from build123d import *

# Parameters (mm, degrees)
SKETCH_1_R          = 1.75
SKETCH_1_R_2        = 7.5
EXTRUDE_1_DEPTH     = 5
SKETCH_1_3_R        = 7.5
SKETCH_1_3_R_2      = 4
EXTRUDE_2_DEPTH     = 24
SKETCH_2_R          = 3
CUT_EXTRUDE_1_DEPTH = 3.1
CHAMFER_1_SIZE      = 0.5
CHAMFER_2_SIZE      = 0.5
FILLET_1_R          = 0.5


with BuildPart() as part:
    # 草图1 → 凸台-拉伸1 (new body)
    with BuildSketch(Plane(origin=(0, 0, 0), x_dir=(1, 0, 0), z_dir=(0, 1, 0))):
        with BuildLine():
            ThreePointArc((-12.5, -9.987492178), (-11.313708499, -11.313708499), (-9.987492178, -12.5))
            Line((-9.987492178, -12.5), (9.987492178, -12.5))
            ThreePointArc((9.987492178, -12.5), (11.313708499, -11.313708499), (12.5, -9.987492178))
            Line((12.5, -9.987492178), (12.5, 9.987492178))
            ThreePointArc((12.5, 9.987492178), (11.313708499, 11.313708499), (9.987492178, 12.5))
            Line((9.987492178, 12.5), (-9.987492178, 12.5))
            ThreePointArc((-9.987492178, 12.5), (-11.313708499, 11.313708499), (-12.5, 9.987492178))
            Line((-12.5, 9.987492178), (-12.5, -9.987492178))
        make_face()
        with Locations((-8.485281374, -8.485281374)):
            Circle(SKETCH_1_R, mode=Mode.SUBTRACT)
        with Locations((8.485281374, -8.485281374)):
            Circle(SKETCH_1_R, mode=Mode.SUBTRACT)
        with Locations((-8.485281374, 8.485281374)):
            Circle(SKETCH_1_R, mode=Mode.SUBTRACT)
        Circle(SKETCH_1_R_2, mode=Mode.SUBTRACT)
        with Locations((8.485281374, 8.485281374)):
            Circle(SKETCH_1_R, mode=Mode.SUBTRACT)
    extrude(amount=EXTRUDE_1_DEPTH)

    # 草图1<3> → 凸台-拉伸2 (add)
    with BuildSketch(Plane(origin=(0, 0, 0), x_dir=(1, 0, 0), z_dir=(0, 1, 0))):
        Circle(SKETCH_1_3_R)
        Circle(SKETCH_1_3_R_2, mode=Mode.SUBTRACT)
    extrude(amount=EXTRUDE_2_DEPTH)

    # 草图2 → 切除-拉伸1 (cut)
    with BuildSketch(Plane.XZ):
        with Locations((-8.485281374, 8.485281374)):
            Circle(SKETCH_2_R)
        with Locations((8.485281374, 8.485281374)):
            Circle(SKETCH_2_R)
        with Locations((8.485281374, -8.485281374)):
            Circle(SKETCH_2_R)
        with Locations((-8.485281374, -8.485281374)):
            Circle(SKETCH_2_R)
    extrude(amount=-CUT_EXTRUDE_1_DEPTH, mode=Mode.SUBTRACT)

    # 倒角1
    chamfer_1_edges = [part.edges().sort_by_distance(p)[0] for p in [
        (0, 5, 12.5),
        (11.313708499, 5, 11.313708499),
        (12.5, 5, 0),
        (11.313708499, 5, -11.313708499),
        (0, 5, -12.5),
        (-11.313708499, 5, -11.313708499),
        (-12.5, 5, 0),
        (-11.313708499, 5, 11.313708499),
    ]]
    chamfer(chamfer_1_edges, length=CHAMFER_1_SIZE)

    # 倒角2
    chamfer_2_edges = [part.edges().sort_by_distance(p)[0] for p in [
        (-11.313708499, 0, 11.313708499),
        (-12.5, 0, 0),
        (-11.313708499, 0, -11.313708499),
        (0, 0, -12.5),
        (11.313708499, 0, -11.313708499),
        (12.5, 0, 0),
        (11.313708499, 0, 11.313708499),
        (0, 0, 12.5),
    ]]
    chamfer(chamfer_2_edges, length=CHAMFER_2_SIZE)

    # 圆角1
    fillet_1_edges = [part.edges().sort_by_distance(p)[0] for p in [
        (-7.5, 24, 0),
    ]]
    fillet(fillet_1_edges, radius=FILLET_1_R)


solid = part.part
Design review of the part built by this model. Coordinates are the model's own, in mm. A direction names the side the tool comes from. Round coordinates to 2 decimals unless told otherwise and drop trailing zeros. Write each loop counter-clockwise with the first axis right and the second up, starting at its lowest first coordinate (ties: lowest second). Pieces come first, ordered by that corner, then holes. Notation, with made-up numbers: M -1.5,-34 L 32.5,-34 A25 cw 32.5,-12 Z; hole C 25.25,-35 d10. An arc over 180 degrees is marked long. One line per item, written item: value. Start each with the question number.
1. Take a section at A-A on x = 0. State the section outline as (y, z) points, then the cut area to 3 significant figures.
2. Take a section at C-C on y = 6.25. State the section outline as (x, z) points.
3. Clearance check with flat-ended pins moving along their axes: P1, Ø1, axis at y = 9.5, z = -6.5, coming from the -X side; P2, Ø1.8, axis at x = 9, z = 7.5, coming from the -Y side; P3, Ø8, axis at y = 14.5, z = 8.5, coming from the -X side; P4, Ø7, axis at x = 0, z = 0, coming from the -Y side. State where each tip first meets the part, or that it passes through.
4. For faces 1 (the face through (6.105, 1.528, -10.311)), 2 (the face through (-8.71, 4.04, 6.75)), list the 3-axis set-ups (+Z, -Z, +X, -X, +Y, -Y) from which the entire face can be reached by the end or side of a thin tool; tool diameter is ignored.
5. Take a section at B-B on z = 0. State the section outline as (x, y) points, then the cut area to 3 significant figures.
6. Draft analysis for pull direction X (two halves, no side actions). For faces 3 (the face through (11.157, 4.746, -11.122)), 4 (the face through (-11.157, 4.746, 11.122)), 5 (the face through (-7, 3.1, -10)), 6 (the face through (0, 2, 12.5)), state which applies: pulls with the +X half, pulls with the -X half, needs draft (parallel to the pull), parting line crosses it, or undercut.
7. To check wall thickness, follow probe 1 along X at (y, z) = (4.5, 9.25); probe 2 along Z at (x, y) = (-8, 3.25); probe 3 along Z at (x, y) = (-0.25, 13). State the ranges of each line that lie inside material, in increasing order. Write a range as from..to.
Computed:
1. outline: M 0,-12 L 0.5,-12.5 L 4.5,-12.5 L 5,-12 L 5,-7.5 L 23.5,-7.5 A0.5 ccw 24,-7 L 24,-4 L 0,-4 Z; M 0,4 L 24,4 L 24,7 A0.5 ccw 23.5,7.5 L 5,7.5 L 5,12 L 4.5,12.5 L 0.5,12.5 L 0,12 Z
1. area: 217 mm²
2. outline: C 0,0 d15; hole C 0,0 d8
3. P1: stops at x = -4.5
3. P2: stops at y = 3.1
3. P3: stops at x = -6
3. P4: passes through
4. face 1: -Y
4. face 2: +Y, -Y
5. outline: M -12.5,0.5 L -12,0 L -4,0 L -4,24 L -7,24 A0.5 ccw -7.5,23.5 L -7.5,5 L -12,5 L -12.5,4.5 Z; M 4,0 L 12,0 L 12.5,0.5 L 12.5,4.5 L 12,5 L 7.5,5 L 7.5,23.5 A0.5 ccw 7,24 L 4,24 Z
5. area: 217 mm²
6. face 3: pulls with the +X half
6. face 4: pulls with the -X half
6. face 5: undercut
6. face 6: needs draft
7. probe 1: x = -12.5..-10.06, -6.91..6.91, 10.06..12.5
7. probe 2: z = -12.5..-10.17, -6.8..6.8, 10.17..12.5
7. probe 3: z = -7.5..-3.99, 3.99..7.5
